Model file for the job. Use its own axes, mm. A direction names the side the tool comes from. Round coordinates to 2 decimals unless told otherwise and drop trailing zeros. Write each loop counter-clockwise with the first axis right and the second up, starting at its lowest first coordinate (ties: lowest second). Pieces come first, ordered by that corner, then holes.
```python
from build123d import *

# Parameters (mm, degrees)
BOSS_EXTRUDE2_DEPTH = 20
SHELL1_T            = -1
SKETCH5_R           = 2.554490716
CUT_EXTRUDE1_DEPTH  = 40.64
SKETCH6_R           = 2.564818337
SKETCH6_R_2         = 2.573203383
SKETCH6_R_3         = 2.511002724
CUT_EXTRUDE3_DEPTH  = 10
SKETCH7_R           = 2.582908473
CUT_EXTRUDE4_DEPTH  = 10
SKETCH9_R           = 2.619720314
CUT_EXTRUDE6_DEPTH  = 10
SKETCH10_R          = 1.6
CUT_EXTRUDE7_DEPTH  = 10


with BuildPart() as part:
    # Sketch1 → Boss-Extrude2 (new body)
    with BuildSketch(Plane(origin=(0, 0, 0), x_dir=(1, 0, 0), z_dir=(0, 1, 0))):
        Polygon((543.066064215, -1022.739016237), (543.066064215, -1018.517703014), (584.976064215, -1018.517703014), (584.976064215, -1056.617703014), (559.865211068, -1056.617703014), (559.865211068, -1096.973737777), (584.842442734, -1096.973737777), (584.842442734, -1103.207715654), (584.842442734, -1135.073737777), (542.932442734, -1135.073737777), (542.932442734, -1128.271846788), (542.932442734, -1095.03316), (504.832442734, -1095.03316), (504.832442734, -1128.271846788), (504.832442734, -1133.999106761), (484.512442734, -1133.999106761), (484.512442734, -1020.023649765), (504.966064215, -1020.023649765), (504.966064215, -1022.739016237), (504.966064215, -1055.977703024), (543.066064215, -1055.977703024), align=None)
    extrude(amount=BOSS_EXTRUDE2_DEPTH)

    # Shell1
    shell1_openings = [part.faces().sort_by_distance(p)[0] for p in [
        (534.165694699, 20, 1076.58641914),
    ]]
    offset(amount=SHELL1_T, openings=shell1_openings, kind=Kind.INTERSECTION)

    # Sketch5 → Cut-Extrude1 (cut)
    with BuildSketch(Plane.XY.offset(1095.03316)):
        with Locations((519.077633691, 10.743789128)):
            Circle(SKETCH5_R)
    extrude(amount=-CUT_EXTRUDE1_DEPTH, mode=Mode.SUBTRACT)

    # Sketch6 → Cut-Extrude3 (cut)
    with BuildSketch(Plane(origin=(584.976064215, 0, 0), x_dir=(0, 0, -1), z_dir=(1, 0, 0))):
        with Locations(Location((-1113.44316001, 10, 0), (0, 0, 180))):
            Circle(SKETCH6_R)
        with Locations((-1075.505431512, 10)):
            Circle(SKETCH6_R_2)
        with Locations((-1037.567703014, 10)):
            Circle(SKETCH6_R_3)
    extrude(amount=-CUT_EXTRUDE3_DEPTH, mode=Mode.SUBTRACT)

    # Sketch7 → Cut-Extrude4 (cut)
    with BuildSketch(Plane(origin=(559.865211068, 0, 0), x_dir=(0, 0, -1), z_dir=(1, 0, 0))):
        with Locations((-1075.505431512, 10)):
            Circle(SKETCH7_R)
    extrude(amount=-CUT_EXTRUDE4_DEPTH, mode=Mode.SUBTRACT)

    # Sketch9 → Cut-Extrude6 (cut)
    with BuildSketch(Plane(origin=(584.842442734, 0, 0), x_dir=(0, 0, -1), z_dir=(1, 0, 0))):
        with Locations((-1113.44316001, 10)):
            Circle(SKETCH9_R)
    extrude(amount=-CUT_EXTRUDE6_DEPTH, mode=Mode.SUBTRACT)

    # Sketch10 → Cut-Extrude7 (cut)
    with BuildSketch(Plane(origin=(0, 1, 0), x_dir=(1, 0, 0), z_dir=(0, 1, 0))):
        with Locations(Location((494.947633691, -1112.763160005, 0), (0, 0, 270))):
            Circle(SKETCH10_R)
        with Locations(Location((550.205220573, -1112.763160005, 0), (0, 0, 270))):
            Circle(SKETCH10_R)
        with Locations(Location((522.30969217, -1084.732316133, 0), (0, 0, 270))):
            Circle(SKETCH10_R)
        with Locations(Location((522.30969217, -1065.102492134, 0), (0, 0, 270))):
            Circle(SKETCH10_R)
        with Locations(Location((550.205220573, -1036.067482908, 0), (0, 0, 270))):
            Circle(SKETCH10_R)
        with Locations(Location((494.023662931, -1036.067482908, 0), (0, 0, 270))):
            Circle(SKETCH10_R)
    extrude(amount=-CUT_EXTRUDE7_DEPTH, mode=Mode.SUBTRACT)


solid = part.part
```
1) Pull direction Z, two halves, no side cores. Call faces 1 (the face through (524, 10, 1095.033)), 2 (the face through (572, 10, 1055.618)), 3 (the face through (584.842, 9.9, 1116.3)), 4 (the face through (583.842, 10.4, 1116.3)): released by +Z, released by -Z, zero draft, split by the parting line, or undercut.
2) Cut at A-A on z = 1049.5. List the corners of the cut face in (x, y).
3) Flat gauge pins, fed straight in: pin 1 Ø6 at (x, y) = (492.5, 12.5) entering from +Z; pin 2 Ø12 at (x, y) = (508.5, 11) entering from -Z; pin 3 Ø3 at (x, z) = (502.5, 1074) entering from +Y; pin 4 Ø1.9 at (x, z) = (522.31, 1065.1) entering from +Y. Where does each tip first touch, or does it go through?
4) Cut at C-C on z = 1071. List the corners of the cut face in (x, y).
5) Cut at B-B on x = 511. List the corners of the cut face in (y, z), and give its area (3 significant figures).
6) Wall check: probe 1 along X at (y, z) = (2.75, 1047.5); probe 2 along X at (y, z) = (5.25, 1096); probe 3 along X at (y, z) = (8.25, 1069). Give the ranges that are in metal, low to high.
7) Which spindle directions (+Z, -Z, +X, -X, +Y, -Y) get a long thin tool onto all of the face, cutting with end or side? Do faces 5 (the face through (559.37, 9.01, 1073.12)), 6 (the face through (572, 10, 1096.974)), 7 (the face through (503.966, 10, 1039)). Say none if no direction does.
Result sheet:
1. face 1: released by +Z
1. face 2: undercut
1. face 3: zero draft
1. face 4: undercut
2. outline: (484.51, 0) - (504.97, 0) - (504.97, 20) - (503.97, 20) - (503.97, 1) - (485.51, 1) - (485.51, 20) - (484.51, 20) - close; (543.07, 0) - (584.98, 0) - (584.98, 20) - (583.98, 20) - (583.98, 1) - (544.07, 1) - (544.07, 20) - (543.07, 20) - close
3. pin 1: stops at z = 1134
3. pin 2: stops at z = 1020.02
3. pin 3: stops at y = 1
3. pin 4: passes through
4. outline: (484.51, 0) - (559.87, 0) - (559.87, 20) - (558.87, 20) - (558.87, 1) - (485.51, 1) - (485.51, 20) - (484.51, 20) - close
5. outline: (0, 1055.98) - (20, 1055.98) - (20, 1056.98) - (1, 1056.98) - (1, 1094.03) - (20, 1094.03) - (20, 1095.03) - (0, 1095.03) - close
5. area: 77.1 mm2
6. probe 1: x = 484.51 to 485.51, 503.97 to 504.97, 543.07 to 544.07, 583.98 to 584.98
6. probe 2: x = 484.51 to 485.51, 503.83 to 504.83, 542.93 to 543.93, 558.87 to 559.87
6. probe 3: x = 484.51 to 485.51, 558.87 to 559.87
7. face 5: +X
7. face 6: +X, +Y, -Y
7. face 7: +Y
